from build123d import *

# Parameters (mm, degrees)
CIRCLE008_R        = 5
EXTRUSION037_DEPTH = 6.500001
RECTANGLE020_W     = 5
RECTANGLE020_H     = 5
EXTRUSION036_DEPTH = 6.500001


with BuildPart() as extrusion037:
    # Circle008 (on Extrusion) → Extrusion037 (new body)
    with BuildSketch(Plane(origin=(-761.714853, -17.774575, 1.366052), x_dir=(0, -1, 0), z_dir=(-1, 0, 0))):
        Circle(CIRCLE008_R)
    extrude(amount=-EXTRUSION037_DEPTH)


with BuildPart() as cut004006005004002008019023005025018:
    # Rectangle020 (on Cut) → Extrusion036 (new body)
    with BuildSketch(Plane(origin=(-755.214852, -17.774575, -3.633948), x_dir=(0, 1, 0), z_dir=(1, 0, 0))):
        with Locations((2.5, 2.5)):
            Rectangle(RECTANGLE020_W, RECTANGLE020_H)
    extrude(amount=-EXTRUSION036_DEPTH)

    # Cut004006005004002008019023005025018: cut Extrusion037
    add(extrusion037.part, mode=Mode.SUBTRACT)


solid = cut004006005004002008019023005025018.part
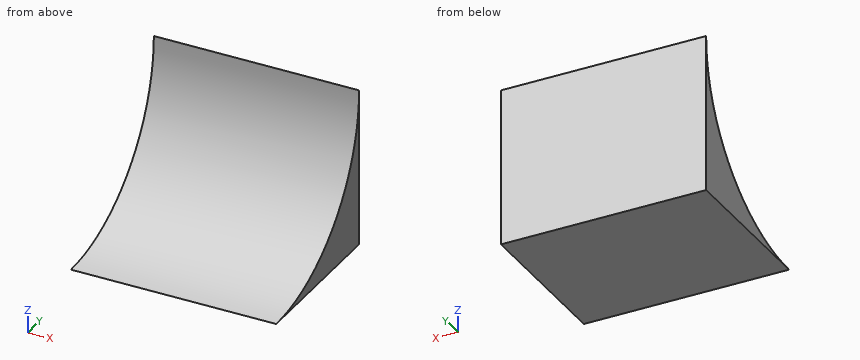
Input: part model. Units: mm. Frame: model coordinates. Give positions to 0.01 mm unless a question says otherwise; leave off trailing zeros. Order: outer loops, then holes, each group sorted by start corner. A loop starts at its lowest first (then second) coordinate and runs counter-clockwise, first axis right, second up. Notation, with made-up numbers: (-29.75, 13) - (-21.75, 13) arc R17 cw to (-21.75, 33) - close; hole circle Ø6 at (36.5, 25.5). An arc over 180 degrees is marked (long way). Write each question's results on one line, items separated by ' | '.
Item 1: Section C-C (y = -14.9). Return loops of the section in (x, z), and give its area (3 significant figures).
A:
outline: (-761.71, -3.63) - (-755.21, -3.63) - (-755.21, -2.73) - (-761.71, -2.73) - close | area: 5.91 mm^2
Item 2: Contact query for flat-ended pins moving along their axis: pin 1 Ø3 at (x, z) = (-758.5, -1.5) entering from -Y; pin 2 Ø2 at (y, z) = (-15.5, -1.5) entering from +X. Output: stop coordinate, or through.
A:
pin 1: stops at y = -15.34 | pin 2: passes through
Item 3: Material intervals for line 1 along Z through (x, y) = (-756.25, -15.35); line 2 along Y through (x, z) = (-760.75, -0.75); line 3 along Z through (x, y) = (-756.75, -16.2), sorted ascending.
A:
line 1: z = -3.63 to -3.01 | line 2: y = -13.24 to -12.77 | line 3: z = -3.63 to -3.38
Item 4: Section A-A (x = -758.25). Return loops of the section in (y, z).
A:
outline: (-17.77, -3.63) - (-12.77, -3.63) - (-12.77, 1.37) arc R5 cw to start
Item 5: Section B-B (z = -1.65). Return loops of the section in (x, y), and give its area (3 significant figures).
A:
outline: (-761.71, -13.79) - (-755.21, -13.79) - (-755.21, -12.77) - (-761.71, -12.77) - close | area: 6.58 mm^2
